from build123d import *

# Parameters (mm, degrees)
SKETCH2_W          = 203.2
SKETCH2_H          = 152.4
LINK2_DEPTH        = 76.2
SKETCH3_R          = 25.4
CUT_EXTRUDE1_DEPTH = 25.4
SKETCH4_W          = 127
SKETCH4_H          = 25.4
CUT_EXTRUDE2_DEPTH = 177.8


with BuildPart() as part:
    # Sketch2 → link2 (new body)
    with BuildSketch(Plane(origin=(0, 0, 0), x_dir=(1, 0, 0), z_dir=(0, 1, 0))):
        Rectangle(SKETCH2_W, SKETCH2_H)
    extrude(amount=LINK2_DEPTH)

    # Sketch3 → Cut-Extrude1 (cut)
    with BuildSketch(Plane.XZ):
        with Locations(Location((50.8, 0, 0), (0, 0, 270))):
            Circle(SKETCH3_R)
    extrude(amount=-CUT_EXTRUDE1_DEPTH, mode=Mode.SUBTRACT)

    # Sketch4 → Cut-Extrude2 (cut)
    with BuildSketch(Plane.ZY.offset(101.6)):
        with Locations((0, 50.8)):
            Rectangle(SKETCH4_W, SKETCH4_H)
    extrude(amount=-CUT_EXTRUDE2_DEPTH, mode=Mode.SUBTRACT)


solid = part.part
Geometry: final body of the model. Coordinates: model frame, mm. A direction names the side the tool comes from. Round coordinates to 2 decimals unless told otherwise and drop trailing zeros. Order: outer loops, then holes, each group sorted by start corner. A loop starts at its lowest first (then second) coordinate and runs counter-clockwise, first axis right, second up. Notation, with made-up numbers: (89.5, 61) - (99.5, 61) arc R17 ccw to (99.5, 81) - close; hole circle Ø5 at (69, 8.5). An arc over 180 degrees is marked (long way). Write each question's results on one line, items separated by ' | '.
Item 1: Reachability of faces 1 (the cylindrical face through (75.984, 12.522, 3.307)), 2 (the flat face through (-1, 38, -76.2)), 3 (the flat face through (76.2, 51, -1)) from +Z, -Z, +X, -X, +Y, -Y: full face, straight path, thin tool, end or side. Return the list, or none.
Completed:
face 1: -Y | face 2: -Z, +X, -X, +Y, -Y | face 3: -X
Item 2: First-contact query: pin 1 Ø1 at (x, z) = (68.5, -45) entering from -Y; pin 2 Ø12 at (y, z) = (53.5, 44.5) entering from -X. Flat tips, straight axial feed; report the tip coordinate or a pass-through.
Completed:
pin 1: y = 0 | pin 2: x = 76.2
Item 3: Section A-A, the plane x = 19.5. Return the cut outline in (y, z).
Completed:
outline: (0, -76.2) - (76.2, -76.2) - (76.2, 76.2) - (0, 76.2) - close; hole (38.1, -63.5) - (63.5, -63.5) - (63.5, 63.5) - (38.1, 63.5) - close
Item 4: Section D-D, the plane y = 21. Return the cut outline in (x, z), and give its area (3 significant figures).
Completed:
outline: (-101.6, -76.2) - (101.6, -76.2) - (101.6, 76.2) - (-101.6, 76.2) - close; hole circle Ø50.8 at (50.8, 0) | area: 28,900 mm^2
Item 5: Section C-C, the plane z = 0. Return the cut outline in (x, y), and give its area (3 significant figures).
Completed:
outline: (-101.6, 0) - (25.4, 0) - (25.4, 25.4) - (76.2, 25.4) - (76.2, 0) - (101.6, 0) - (101.6, 76.2) - (-101.6, 76.2) - (-101.6, 63.5) - (76.2, 63.5) - (76.2, 38.1) - (-101.6, 38.1) - close | area: 9,680 mm^2
Item 6: Section B-B, the plane y = 44. Return the cut outline in (x, z), and give its area (3 significant figures).
Completed:
outline: (-101.6, -76.2) - (101.6, -76.2) - (101.6, 76.2) - (-101.6, 76.2) - (-101.6, 63.5) - (76.2, 63.5) - (76.2, -63.5) - (-101.6, -63.5) - close | area: 8,390 mm^2
Item 7: Material intervals for line 1 along Y through (x, z) = (-57.5, -21); line 2 along Z through (x, y) = (50, 11); line 3 along Z through (x, y) = (-18.5, 46.5), sorted ascending. Write a range as [from, to].
Completed:
line 1: [0, 38.1], [63.5, 76.2] | line 2: [-76.2, -25.39], [25.39, 76.2] | line 3: [-76.2, -63.5], [63.5, 76.2]
Item 8: Mould query, pull axis Y, two halves, no side actions, for faces 4 (the flat face through (-1, 76.2, -1)), 5 (the flat face through (-14, 63.5, -1)), 6 (the flat face through (-1, 38, 76.2)). Classes: pulls with the +Y half, pulls with the -Y half, needs draft (parallel to the pull), parting line crosses it, or undercut.
Completed:
face 4: pulls with the +Y half | face 5: undercut | face 6: needs draft
